Build history of the part. All positions in model axes, mm. A direction names the side the tool comes from. Round coordinates to 2 decimals unless told otherwise and drop trailing zeros. Loops run counter-clockwise (first coordinate to the right, second up) from the corner with the lowest first, then second, coordinate; pieces in that order, holes last. Notation, with made-up numbers: M 26.25,70 L 42.25,70 A25 ccw 42.25,106 Z; hole C 85,70.5 d9. An arc over 180 degrees is marked long. One line per item, written item: value.
```python
from build123d import *

# Parameters (mm, degrees)
F1_DEPTH = 25


# Not quite as in the source:
# - a feature names something its author has since deleted; it is built from what else it names


with BuildPart() as f1:
    # F0 (on Front) → F1 (new body)
    with BuildSketch(Plane.XZ):
        with BuildLine():
            Line((-10, -5.576437097), (10, -5.576437097))
            Line((10, -5.576437097), (10, -2.201012618))
            Line((10, -2.201012618), (9.4, -1.8546024565))
            Line((9.4, -1.8546024565), (9.4, 0.3245011641))
            Line((9.4, 0.3245011641), (10, 0.6709113256))
            Line((10, 0.6709113256), (10, 5.576437097))
            Line((10, 5.576437097), (2.2236531144, 5.576437097))
            ThreePointArc((2.2236531144, 5.576437097), (2.7991926821, 4.6417723907), (3, 3.5626429599))
            ThreePointArc((3, 3.5626429599), (-1.0791294308, 0.7634502778), (-2.2236531144, 5.576437097))
            Line((-2.2236531144, 5.576437097), (-10, 5.576437097))
            Line((-10, 5.576437097), (-10, 0.6884473353))
            Line((-10, 0.6884473353), (-8.6999533325, 1.4390296287))
            Line((-8.6999533325, 1.4390296287), (-6.7999051139, 0.3420362782))
            Line((-6.7999051139, 0.3420362782), (-6.7999051139, -1.8519504229))
            Line((-6.7999051139, -1.8519504229), (-8.6999533325, -2.9489437734))
            Line((-8.6999533325, -2.9489437734), (-10, -2.19836148))
            Line((-10, -2.19836148), (-10, -5.576437097))
        make_face()
        Polygon((10, 0.6709113256), (10, -2.201012618), (11.2871590928, -2.9441542667), (13.1743181857, -1.8546024565), (13.1743181857, 0.3245011641), (11.2871590928, 1.4140529743), align=None)
        Polygon((9.4, -1.8546024565), (10, -2.201012618), (10, 0.6709113256), (9.4, 0.3245011641), align=None)
    extrude(amount=F1_DEPTH)


solid = f1.part
```
Item 1: Slice it at C-C, the plane z = -4. Give the cut face in (x, y), and give its area (3 significant figures).
Check values:
outline: M -10,-25 L 10,-25 L 10,0 L -10,0 Z
area: 500 mm2
Item 2: Slice it at B-B, the plane y = -15.25. Give the cut face in (x, z), and give its area (3 significant figures).
Check values:
outline: M -10,-5.58 L 10,-5.58 L 10,-2.2 L 11.29,-2.94 L 13.17,-1.85 L 13.17,0.32 L 11.29,1.41 L 10,0.67 L 10,5.58 L 2.22,5.58 A3 cw long -2.22,5.58 L -10,5.58 L -10,0.69 L -8.7,1.44 L -6.8,0.34 L -6.8,-1.85 L -8.7,-2.95 L -10,-2.2 Z
area: 198 mm2
Item 3: Pull direction Z, two halves, no side cores. Call faces 1 (the face through (10.635, -12.325, -2.567)), 2 (the face through (-7.763, -12.325, 0.898)), 3 (the face through (6, -12, 5.576)): pulls with the +Z half, pulls with the -Z half, needs draft (parallel to the pull), parting line crosses it, or undercut.
Check values:
face 1: pulls with the -Z half
face 2: undercut
face 3: pulls with the +Z half
Item 4: Slice it at A-A, the plane z = 3. Give the cut face in (x, y).
Check values:
outline: M -10,-25 L -2.95,-25 L -2.95,0 L -10,0 Z; M 2.95,-25 L 10,-25 L 10,0 L 2.95,0 Z
Item 5: Drop a flat-ended pin along its axis: P1, Ø3.5, axis at y = -8, z = -4, coming from the +X side. Give the stop position or say it passes through.
Check values:
P1: stops at x = 12.49
Item 6: Slice it at D-D, the plane x = 0. Give the cut face in (y, z), and give its area (3 significant figures).
Check values:
outline: M -25,-5.58 L 0,-5.58 L 0,0.56 L -25,0.56 Z
area: 153 mm2
Item 7: Wall check: line 1 along X through (y, z) = (-8.5, 3.5); line 2 along X through (y, z) = (-23.5, -0.5); line 3 along Z through (x, y) = (0, -18.5). Give the ranges that are in metal, low to high.
Check values:
line 1: x = -10 to -3, 3 to 10
line 2: x = -6.8 to 13.17
line 3: z = -5.58 to 0.56
Item 8: Which spindle directions (+Z, -Z, +X, -X, +Y, -Y) get a long thin tool onto all of the face, cutting with end or side? Do faces 4 (the face through (10, -12, -4)), 5 (the face through (-9.36, -12.32, 1.06)), 6 (the face through (-6.8, -12, -1)), 7 (the face through (10.653, -12.325, 1.048)), 8 (the face through (1, 0, 0)). Say none if no direction does.
Check values:
face 4: -Z, +Y, -Y
face 5: +Y, -Y
face 6: -X, +Y, -Y
face 7: +Z, +Y, -Y
face 8: +Z, -Z, +X, -X, +Y
